Check sheet for the modelled part. Datum: model origin and axes. Units: mm. A direction names the side the tool comes from. Round coordinates to 2 decimals unless told otherwise and drop trailing zeros. Write each loop counter-clockwise with the first axis right and the second up, starting at its lowest first coordinate (ties: lowest second). Pieces come first, ordered by that corner, then holes. Notation, with made-up numbers: M -28.75,-17.75 L -2.75,-17.75 A26 cw -2.75,18.25 Z; hole C 60.25,49.5 d10. An arc over 180 degrees is marked long. Put each result on its own line as item: value.
```python
from build123d import *

# Parameters (mm, degrees)
BOSS_EXTRUDE1_DEPTH = 3.5
SKETCH4_OUTSIDE_W   = 88.856
SKETCH4_OUTSIDE_H   = 90.094
SKETCH4_OUTSIDE_R   = 4
CUT_EXTRUDE1_DEPTH  = 21.434855843
CUT_EXTRUDE1_DRAFT  = -60


with BuildPart() as part:
    # Sketch2 → Revolve1 (revolve)
    with BuildSketch(Plane(origin=(0, 0, 0), x_dir=(0, 0, -1), z_dir=(1, 0, 0)), mode=Mode.PRIVATE) as revolve1_sk:
        Polygon((-9.75, 4), (-9.75, 0), (9.75, 0), (9.75, 1.9), (9.15, 2.5), (-6.25, 2.5), (-6.25, 4), align=None)
    revolve(revolve1_sk.sketch.rotate(Axis((0, 0, 9.75), (0, 0, -1)), 90), axis=Axis((0, 0, 9.75), (0, 0, -1)))

    # Sketch3 → Boss-Extrude1 (add)
    with BuildSketch(Plane.XY.offset(9.75)):
        Polygon((0, 4.618802154), (-4, 2.309401077), (-4, -2.309401077), (0, -4.618802154), (4, -2.309401077), (4, 2.309401077), align=None)
    extrude(amount=-BOSS_EXTRUDE1_DEPTH)


with BuildPart() as cut_extrude1_tool:
    # Sketch4 outside → Cut-Extrude1 (with draft: the straight prism first)
    with BuildSketch(Plane.XY.offset(9.75)):
        Rectangle(SKETCH4_OUTSIDE_W, SKETCH4_OUTSIDE_H)
        Circle(SKETCH4_OUTSIDE_R, mode=Mode.SUBTRACT)
    extrude(amount=-CUT_EXTRUDE1_DEPTH)
    # Cut-Extrude1: the draft: its side faces are tilted about the plane it starts from
    cut_extrude1_sides = [cut_extrude1_tool.faces().sort_by_distance(p)[0] for p in [
        (0, -45.047, -0.967427922),
        (44.428, 0, -0.967427922),
        (0, 45.047, -0.967427922),
        (-44.428, 0, -0.967427922),
        (-4, 0, -0.967427922),
    ]]
    draft(cut_extrude1_sides, Plane.XY.offset(9.75), CUT_EXTRUDE1_DRAFT)


with BuildPart() as part_1:
    add(part.part)

    # Cut-Extrude1: cut by cut_extrude1_tool
    add(cut_extrude1_tool.part, mode=Mode.SUBTRACT)


solid = part_1.part
```
1. Cross-section at A-A (z = -8). Enter the section's corners in (x, y), then the cut area to 3 significant figures.
Computed values:
outline: C 0,0 d5
area: 19.6 mm2
2. Scan lines: probe 1 along Z at (x, y) = (3, -0.75); probe 2 along X at (y, z) = (1.5, -8.25); probe 3 along X at (y, z) = (-1.75, -0.5). Record each from-to range of solid material in increasing order.
Computed values:
probe 1: z = 6.25 to 9.75
probe 2: x = -2 to 2
probe 3: x = -1.79 to 1.79
3. Access from +Z, -Z, +X, -X, +Y, -Y to the whole of each face (thin tool, end or side, straight path). Record for faces 1 (the flat face through (2, -2, 6.25)), 2 (the flat face through (0, 0, 9.75)).
Computed values:
face 1: -Z
face 2: +Z, +X, -X, +Y, -Y
4. Depth check by flat-ended pin: pin 1 Ø4 at (y, z) = (-1.5, -2) entering from +X; pin 2 Ø4 at (y, z) = (0.5, 0) entering from -X; pin 3 Ø3 at (x, z) = (-2.5, 7.5) entering from +Y. Enter the tip coordinate at first touch or a pass-through.
Computed values:
pin 1: stops at x = 2.5
pin 2: stops at x = -2.5
pin 3: stops at y = 4.04
